Can you work these out from the model? Positions are in its coordinate system, mm. Face numbers are marked on the shaded views. A direction names the side the tool comes from. Round coordinates to 2 decimals unless told otherwise and drop trailing zeros. Order: outer loops, then holes, each group sorted by start corner. A loop starts at its lowest first (then second) coordinate and runs counter-clockwise, first axis right, second up. Notation, with made-up numbers: (59, -26.75) -> (65, -26.75) arc R14 ccw to (65, -13.75) -> close; hole circle Ø5 at (-5.75, 34.5). An arc over 180 degrees is marked (long way). Use a Markdown table: item, result. Add a question column.
Q1. I need wall thicknesses on line 1 along X through (y, z) = (-2.5, 110); line 2 along Z through (x, y) = (-60.5, 66.5). Which ranges of each line are inside material? Lowest first, please. Write a range as [from, to].
Q2. If we section it at A-A on z = 21.5: List the corners of the cut face in (x, y) for me.
Q3. If we section it at D-D on x = 5.5: List the corners of the cut face in (y, z) for me, plus the area to 3 significant figures.
Q4. If we section it at B-B on x = -58.5: List the corners of the cut face in (y, z) for me.
Q5. For the marked faces 4 and 5, which set-ups out of +Z, -Z, +X, -X, +Y, -Y let a thin tool reach every point of the face, with its end or its side?
Q6. We'd pull the mould along X, two halves only. Please class the marked faces 1, 2 and 3: +X half, -X half, draft (parallel to the pull), parting line (faces both ways), or undercut.
Q7. I'm going to push a flat-ended pin straight in: pin 1 Ø10 at (x, y) = (-27.5, 5.5) entering from +Z. Where does the tip first touch, or does it pass through?
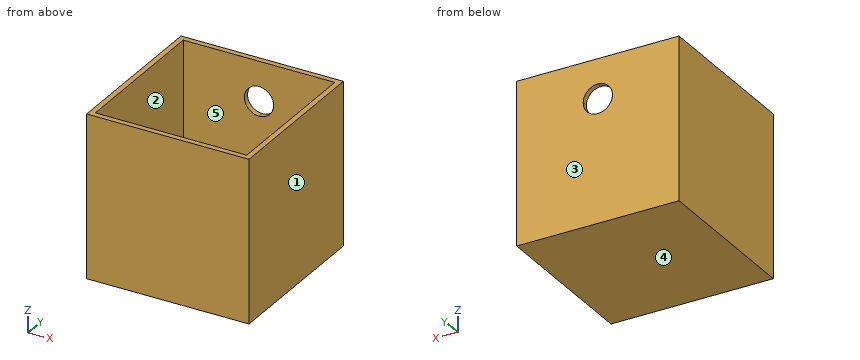
```python
from build123d import *

# Parameters (mm, degrees)
F0_W     = 150
F0_H     = 150
F1_DEPTH = 150
F2_T     = -5
F4_DEPTH = 5


with BuildPart() as f1:
    # F0 (on Top) → F1 (new body)
    with BuildSketch(Plane.XY):
        Rectangle(F0_W, F0_H)
    extrude(amount=F1_DEPTH)

    # F2
    f2_openings = [f1.faces().sort_by_distance(p)[0] for p in [
        (0, 0, 150),
    ]]
    offset(amount=F2_T, openings=f2_openings)

    # F3 (on face) → F4 (cut)
    with BuildSketch(Plane.XZ.offset(-70)):
        with BuildLine():
            ThreePointArc((13.5, 113.5), (9.545942, 123.045942), (0, 127))
            Line((0, 127), (0, 100))
            ThreePointArc((0, 100), (9.545942, 103.954058), (13.5, 113.5))
        make_face()
        with BuildLine():
            Line((0, 100), (0, 127))
            ThreePointArc((0, 127), (-13.5, 113.5), (0, 100))
        make_face()
    extrude(amount=-F4_DEPTH, mode=Mode.SUBTRACT)


solid = f1.part
```
Answer below:
| question | item | result |
|---|---|---|
| 1 | line 1 | [-75, -70], [70, 75] |
| 1 | line 2 | [0, 5] |
| 2 | outline | (-75, -75) -> (75, -75) -> (75, 75) -> (-75, 75) -> close; hole (-70, -70) -> (70, -70) -> (70, 70) -> (-70, 70) -> close |
| 3 | outline | (-75, 0) -> (75, 0) -> (75, 101.17) -> (70, 101.17) -> (70, 5) -> (-70, 5) -> (-70, 150) -> (-75, 150) -> close; (70, 125.83) -> (75, 125.83) -> (75, 150) -> (70, 150) -> close |
| 3 | area | 2,080 mm² |
| 4 | outline | (-75, 0) -> (75, 0) -> (75, 150) -> (70, 150) -> (70, 5) -> (-70, 5) -> (-70, 150) -> (-75, 150) -> close |
| 5 | face 4 | -Z, +X, -X, +Y, -Y |
| 5 | face 5 | +Z |
| 6 | face 1 | +X half |
| 6 | face 2 | undercut |
| 6 | face 3 | draft |
| 7 | pin 1 | z = 5 |
